Part model, mm, in its own coordinate system. Face numbers are marked on the shaded views. A direction names the side the tool comes from. Round coordinates to 2 decimals unless told otherwise and drop trailing zeros. Order: outer loops, then holes, each group sorted by start corner. A loop starts at its lowest first (then second) coordinate and runs counter-clockwise, first axis right, second up. Notation, with made-up numbers: M -12,58 L 21,58 A16 cw 21,89 Z; hole C -9,40.5 d3. An arc over 180 degrees is marked long. Write each question's results on one line, items separated by ' | '. Start each with the question number.
1. Band-saw the part on A-A, the plane y = -36. List the corners of the cut face in (x, z), then the cut area to 3 significant figures.
2. Band-saw the part on B-B, the plane x = 13. List the corners of the cut face in (y, z).
3. Band-saw the part on D-D, the plane y = -21. List the corners of the cut face in (x, z).
4. Drop flat-ended pins along their axis: pin 1 Ø4.5 at (y, z) = (-37.5, -54) entering from +X; pin 2 Ø7.5 at (x, z) = (33, -66.5) entering from +Y. Give the stop position or say it passes through.
5. Which spindle directions (+Z, -Z, +X, -X, +Y, -Y) get a long thin tool onto all of the face, cutting with end or side? Do the marked faces 1, 2 and 3. Say none if no direction does.
6. Probe L1, parallel to Z at x = 3.5, y = -28; L2, parallel to Y at x = 34, z = -34.5; L3, parallel to X at y = -36, z = -11. List the from-to ranges inside material, lowest first. Write a range as [from, to].
7. Band-saw the part on C-C, the plane z = -54.5. List the corners of the cut face in (x, y), then the cut area to 3 significant figures.
8. Two-plate mould, pull along Y, no slides. Class the marked faces 4, 5 and 6: +Y half, -Y half, draft (parallel to the pull), parting line (faces both ways), or undercut.
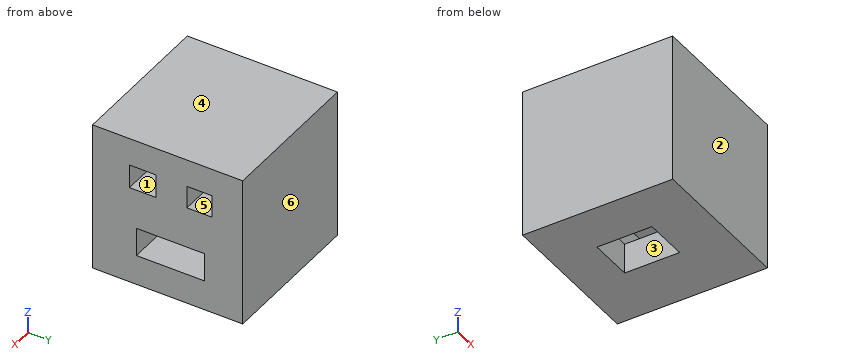
```python
from build123d import *

# Parameters (mm, degrees)
F0_W     = 76.2
F0_H     = 76.2
F1_DEPTH = 76.2
F2_W     = 12.78471
F2_H     = 11.434516
F2_W_2   = 13.372
F2_H_2   = 12.032146
F2_W_3   = 34.573561
F2_H_3   = 14.494572
F4_DEPTH = 73.040023
F3_W     = 22.247531
F3_H     = 27.866135
F5_DEPTH = 72.060369


with BuildPart() as f1:
    # F0 (on Front) → F1 (new body)
    with BuildSketch(Plane.XZ):
        with Locations((38.1, -38.1)):
            Rectangle(F0_W, F0_H)
    extrude(amount=F1_DEPTH)

    # F2 (on face) → F4 (cut)
    with BuildSketch(Plane.YZ.offset(76.2)):
        with Locations((-21.916236, -19.748955)):
            Rectangle(F2_W, F2_H)
        with Locations((-50.78535, -20.083058)):
            Rectangle(F2_W_2, F2_H_2)
        with Locations((-36.654551, -53.62192)):
            Rectangle(F2_W_3, F2_H_3)
    extrude(amount=-F4_DEPTH, mode=Mode.SUBTRACT)

    # F3 (on face) → F5 (cut)
    with BuildSketch(Plane(origin=(0, 0, -76.2), x_dir=(1, 0, 0), z_dir=(0, 0, -1))):
        with Locations((35.47072, 36.344724)):
            Rectangle(F3_W, F3_H)
    extrude(amount=-F5_DEPTH, mode=Mode.SUBTRACT)


solid = f1.part
```
Solution:
1) outline: M 0,-76.2 L 24.35,-76.2 L 24.35,-60.87 L 3.16,-60.87 L 3.16,-46.37 L 24.35,-46.37 L 24.35,-4.14 L 46.59,-4.14 L 46.59,-46.37 L 76.2,-46.37 L 76.2,0 L 0,0 Z; M 46.59,-76.2 L 76.2,-76.2 L 76.2,-60.87 L 46.59,-60.87 Z | area: 3,470 mm^2
2) outline: M -76.2,-76.2 L 0,-76.2 L 0,0 L -76.2,0 Z; hole M -57.47,-26.1 L -44.1,-26.1 L -44.1,-14.07 L -57.47,-14.07 Z; hole M -53.94,-60.87 L -19.37,-60.87 L -19.37,-46.37 L -53.94,-46.37 Z; hole M -28.31,-25.47 L -15.52,-25.47 L -15.52,-14.03 L -28.31,-14.03 Z
3) outline: M 0,-76.2 L 76.2,-76.2 L 76.2,-60.87 L 3.16,-60.87 L 3.16,-46.37 L 76.2,-46.37 L 76.2,-25.47 L 3.16,-25.47 L 3.16,-14.03 L 76.2,-14.03 L 76.2,0 L 0,0 Z
4) pin 1: x = 3.16 | pin 2: y = 0
5) face 1: +X | face 2: +Z, -Z, +X, -X, -Y | face 3: -Z
6) L1: [-76.2, -60.87], [-46.37, -25.47], [-14.03, 0] | L2: [-76.2, -50.28], [-22.41, 0] | L3: [0, 24.35], [46.59, 76.2]
7) outline: M 0,-76.2 L 76.2,-76.2 L 76.2,-53.94 L 3.16,-53.94 L 3.16,-19.37 L 76.2,-19.37 L 76.2,0 L 0,0 Z | area: 3,280 mm^2
8) face 4: draft | face 5: undercut | face 6: +Y half
